Source: CAD feature listing. Evaluate the final solid. Frame: model axes, mm. Face numbers are marked on the shaded views. A direction names the side the tool comes from. Round coordinates to 2 decimals unless told otherwise and drop trailing zeros. Loops run counter-clockwise (first coordinate to the right, second up) from the corner with the lowest first, then second, coordinate; pieces in that order, holes last.
(1) Section C-C, the plane y = -6. Return the cut outline in (x, z), plus the area to 3 significant figures.
(2) Section B-B, the plane x = 42. Return the cut outline in (y, z).
(3) Material intervals for probe 1 along Y at (x, z) = (-63.5, 27.7); probe 2 along Y at (x, z) = (64, 7); probe 3 along Y at (x, z) = (5, 6.5), sorted ascending.
(4) Section D-D, the plane x = 1. Return the cut outline in (y, z).
(5) First-contact query: pin 1 Ø3 at (x, y) = (63, 24.5) entering from +Z; pin 2 Ø3.5 at (x, y) = (-54.5, 26.5) entering from +Z; pin 3 Ø3 at (x, y) = (-8.5, 8) entering from -Z. Flat tips, straight axial feed; report the tip coordinate or a pass-through.
(6) Section A-A, the plane x = -42. Return the cut outline in (y, z), plus the area to 3 significant figures.
(7) Set-up query: the marked faces 4 and 5. Return all of +Z, -Z, +X, -X, +Y, -Y with unobstructed straight access to the full face (end or side cutting, diameter ignored); none if empty.
(8) Mould query, pull axis X, two halves, no side actions, for the marked faces 1, 2 and 3. Classes: pulls with the +X half, pulls with the -X half, needs draft (parallel to the pull), parting line crosses it, or undercut.
```python
from build123d import *

# Parameters (mm, degrees)
SKETCH002_W     = 140
SKETCH002_H     = 66
PAD001_DEPTH    = 4
SKETCH003_W     = 136
SKETCH003_H     = 62
PAD002_DEPTH    = 30
SKETCH004_R     = 3
POCKET001_DEPTH = 5
FILLET_R        = 2
FILLET001_R     = 2
SKETCH005_R     = 1.5
SKETCH005_W     = 10
SKETCH005_H     = 5
POCKET002_DEPTH = 5
SKETCH006_W     = 18
SKETCH006_H     = 9
SKETCH006_W_2   = 9
PAD003_DEPTH    = 6
SKETCH007_W     = 9
SKETCH007_H     = 9
PAD004_DEPTH    = 19
SKETCH008_W     = 9
SKETCH008_H     = 9
PAD005_DEPTH    = 19
SKETCH009_W     = 9
SKETCH009_H     = 9
PAD006_DEPTH    = 25
FILLET004_R     = 1
SKETCH014_W     = 5.5
SKETCH014_H     = 3
POCKET005_DEPTH = 7.5
SKETCH015_W     = 5.5
SKETCH015_H     = 3
POCKET006_DEPTH = 7.5
SKETCH016_W     = 5.5
SKETCH016_H     = 3
POCKET007_DEPTH = 7.4
SKETCH017_W     = 5.5
SKETCH017_H     = 3
POCKET008_DEPTH = 7.5
SKETCH018_W     = 5.5
SKETCH018_H     = 3
POCKET009_DEPTH = 7.5
SKETCH019_W     = 5.5
SKETCH019_H     = 3
POCKET010_DEPTH = 7.5
SKETCH020_R     = 1.6
POCKET011_DEPTH = 12
SKETCH021_R     = 1.6
POCKET012_DEPTH = 12
SKETCH022_R     = 1.6
POCKET013_DEPTH = 12
SKETCH023_R     = 1.6
POCKET014_DEPTH = 12
SKETCH024_R     = 1.6
POCKET015_DEPTH = 8
SKETCH025_R     = 1.6
POCKET016_DEPTH = 8
SKETCH026_R     = 1.6
POCKET017_DEPTH = 8
SKETCH027_R     = 1.6
POCKET018_DEPTH = 8
FILLET005_R     = 1


with BuildPart() as part:
    # Sketch002 → Pad001 (new body)
    with BuildSketch(Plane.XY):
        Rectangle(SKETCH002_W, SKETCH002_H)
    extrude(amount=PAD001_DEPTH)

    # Sketch003 (on Face6 of Pad001) → Pad002 (join)
    with BuildSketch(Plane.XY.offset(4)):
        Polygon((-70, 33), (-70, -33), (-68, -33), (68, -33), (70, -33), (70, 33), (68, 33), (-68, 33), align=None)
        Rectangle(SKETCH003_W, SKETCH003_H, mode=Mode.SUBTRACT)
    extrude(amount=PAD002_DEPTH)

    # Sketch004 (on Face2 of Pad002) → Pocket001 (cut)
    with BuildSketch(Plane.XZ.offset(33)):
        with Locations((42, 25)):
            Circle(SKETCH004_R)
        with Locations((-42, 25)):
            Circle(SKETCH004_R)
        with Locations((-14, 25)):
            Circle(SKETCH004_R)
        with Locations((14, 25)):
            Circle(SKETCH004_R)
    extrude(amount=-POCKET001_DEPTH, mode=Mode.SUBTRACT)

    # Fillet
    fillet_edges = [part.edges().sort_by_distance(p)[0] for p in [
        (-70, -33, 17),
        (70, -33, 17),
    ]]
    fillet(fillet_edges, radius=FILLET_R)

    # Fillet001
    fillet001_edges = [part.edges().sort_by_distance(p)[0] for p in [
        (70, 33, 17),
        (-70, 33, 17),
    ]]
    fillet(fillet001_edges, radius=FILLET001_R)

    # Sketch005 (on Face5 of Fillet001) → Pocket002 (cut)
    with BuildSketch(Plane(origin=(0, 33, 0), x_dir=(-1, 0, 0), z_dir=(0, 1, 0))):
        with Locations((-34.5, 9)):
            Circle(SKETCH005_R)
        with Locations((-51, 9)):
            Circle(SKETCH005_R)
        with Locations((-42.75, 9)):
            Rectangle(SKETCH005_W, SKETCH005_H)
    extrude(amount=-POCKET002_DEPTH, mode=Mode.SUBTRACT)

    # Sketch006 (on Face25 of Pocket002) → Pad003 (join)
    with BuildSketch(Plane.XY.offset(4)):
        with Locations((-59, 26.5)):
            Rectangle(SKETCH006_W, SKETCH006_H)
        with Locations((-59, -26.5)):
            Rectangle(SKETCH006_W, SKETCH006_H)
        with Locations((18.5, 26.5)):
            Rectangle(SKETCH006_W_2, SKETCH006_H)
        with Locations((18.5, -26.5)):
            Rectangle(SKETCH006_W_2, SKETCH006_H)
    extrude(amount=PAD003_DEPTH)

    # Sketch007 (on Face31 of Pad003) → Pad004 (join)
    with BuildSketch(Plane.XY.offset(10)):
        with Locations((-63.5, 26.5)):
            Rectangle(SKETCH007_W, SKETCH007_H)
    extrude(amount=PAD004_DEPTH)

    # Sketch008 (on Face30 of Pad004) → Pad005 (join)
    with BuildSketch(Plane.XY.offset(10)):
        with Locations((-63.5, -26.5)):
            Rectangle(SKETCH008_W, SKETCH008_H)
    extrude(amount=PAD005_DEPTH)

    # Sketch009 (on Face25 of Pad005) → Pad006 (join)
    with BuildSketch(Plane.XY.offset(4)):
        with Locations((63.5, 26.5)):
            Rectangle(SKETCH009_W, SKETCH009_H)
        with Locations((63.5, -26.5)):
            Rectangle(SKETCH009_W, SKETCH009_H)
    extrude(amount=PAD006_DEPTH)

    # Fillet004
    fillet004_edges = [part.edges().sort_by_distance(p)[0] for p in [
        (-68, 31, 31.5),
        (68, 31, 31.5),
        (68, -31, 31.5),
        (-68, -31, 31.5),
    ]]
    fillet(fillet004_edges, radius=FILLET004_R)

    # Sketch014 (on Face36 of Fillet004) → Pocket005 (cut)
    with BuildSketch(Plane.XZ.offset(-22)):
        with Locations((-63.5, 23.5)):
            Rectangle(SKETCH014_W, SKETCH014_H)
        with Locations((-54.5, 6.5)):
            Rectangle(SKETCH014_W, SKETCH014_H)
    extrude(amount=-POCKET005_DEPTH, mode=Mode.SUBTRACT)

    # Sketch015 (on Face33 of Pocket005) → Pocket006 (cut)
    with BuildSketch(Plane.XZ.offset(-22)):
        with Locations((63.5, 23.5)):
            Rectangle(SKETCH015_W, SKETCH015_H)
    extrude(amount=-POCKET006_DEPTH, mode=Mode.SUBTRACT)

    # Sketch016 (on Face35 of Pocket006) → Pocket007 (cut)
    with BuildSketch(Plane(origin=(0, -22, 0), x_dir=(-1, 0, 0), z_dir=(0, 1, 0))):
        with Locations((63.5, 23.5)):
            Rectangle(SKETCH016_W, SKETCH016_H)
        with Locations((54.5, 6.5)):
            Rectangle(SKETCH016_W, SKETCH016_H)
    extrude(amount=-POCKET007_DEPTH, mode=Mode.SUBTRACT)

    # Sketch017 (on Face34 of Pocket007) → Pocket008 (cut)
    with BuildSketch(Plane(origin=(0, -22, 0), x_dir=(-1, 0, 0), z_dir=(0, 1, 0))):
        with Locations((-63.5, 23.5)):
            Rectangle(SKETCH017_W, SKETCH017_H)
    extrude(amount=-POCKET008_DEPTH, mode=Mode.SUBTRACT)

    # Sketch018 (on Face53 of Pocket008) → Pocket009 (cut)
    with BuildSketch(Plane.XZ.offset(-22)):
        with Locations((18.5, 6.5)):
            Rectangle(SKETCH018_W, SKETCH018_H)
    extrude(amount=-POCKET009_DEPTH, mode=Mode.SUBTRACT)

    # Sketch019 (on Face52 of Pocket009) → Pocket010 (cut)
    with BuildSketch(Plane(origin=(0, -22, 0), x_dir=(-1, 0, 0), z_dir=(0, 1, 0))):
        with Locations((-18.5, 6.5)):
            Rectangle(SKETCH019_W, SKETCH019_H)
    extrude(amount=-POCKET010_DEPTH, mode=Mode.SUBTRACT)

    # Sketch020 (on Face37 of Pocket010) → Pocket011 (cut)
    with BuildSketch(Plane.XY.offset(29)):
        with Locations((-63.5, 26.5)):
            Circle(SKETCH020_R)
    extrude(amount=-POCKET011_DEPTH, mode=Mode.SUBTRACT)

    # Sketch021 (on Face18 of Pocket011) → Pocket012 (cut)
    with BuildSketch(Plane.XY.offset(29)):
        with Locations((-63.5, -26.5)):
            Circle(SKETCH021_R)
    extrude(amount=-POCKET012_DEPTH, mode=Mode.SUBTRACT)

    # Sketch022 (on Face32 of Pocket012) → Pocket013 (cut)
    with BuildSketch(Plane.XY.offset(29)):
        with Locations((63.5, 26.5)):
            Circle(SKETCH022_R)
    extrude(amount=-POCKET013_DEPTH, mode=Mode.SUBTRACT)

    # Sketch023 (on Face22 of Pocket013) → Pocket014 (cut)
    with BuildSketch(Plane.XY.offset(29)):
        with Locations((63.5, -26.5)):
            Circle(SKETCH023_R)
    extrude(amount=-POCKET014_DEPTH, mode=Mode.SUBTRACT)

    # Sketch024 (on Face43 of Pocket014) → Pocket015 (cut)
    with BuildSketch(Plane.XY.offset(10)):
        with Locations((-54.5, 26.5)):
            Circle(SKETCH024_R)
    extrude(amount=-POCKET015_DEPTH, mode=Mode.SUBTRACT)

    # Sketch025 (on Face40 of Pocket015) → Pocket016 (cut)
    with BuildSketch(Plane.XY.offset(10)):
        with Locations((18.5, 26.5)):
            Circle(SKETCH025_R)
    extrude(amount=-POCKET016_DEPTH, mode=Mode.SUBTRACT)

    # Sketch026 (on Face26 of Pocket016) → Pocket017 (cut)
    with BuildSketch(Plane.XY.offset(10)):
        with Locations((18.5, -26.5)):
            Circle(SKETCH026_R)
    extrude(amount=-POCKET017_DEPTH, mode=Mode.SUBTRACT)

    # Sketch027 (on Face20 of Pocket017) → Pocket018 (cut)
    with BuildSketch(Plane.XY.offset(10)):
        with Locations((-54.5, -26.5)):
            Circle(SKETCH027_R)
    extrude(amount=-POCKET018_DEPTH, mode=Mode.SUBTRACT)

    # Fillet005
    fillet005_edges = [part.edges().sort_by_distance(p)[0] for p in [
        (68, 22, 16.5),
        (59, 22, 16.5),
        (59, 31, 16.5),
        (23, 31, 7),
        (23, 22, 7),
        (14, 22, 7),
        (14, 31, 7),
        (-68, 22, 16.5),
        (-59, 22, 19.5),
        (-59, 31, 19.5),
        (-50, 22, 7),
        (-50, 31, 7),
        (68, -22, 16.5),
        (59, -22, 16.5),
        (59, -31, 16.5),
        (23, -31, 7),
        (23, -22, 7),
        (14, -22, 7),
        (14, -31, 7),
        (-50, -31, 7),
        (-50, -22, 7),
        (-59, -22, 19.5),
        (-68, -22, 16.5),
        (-59, -31, 19.5),
    ]]
    fillet(fillet005_edges, radius=FILLET005_R)


solid = part.part
```
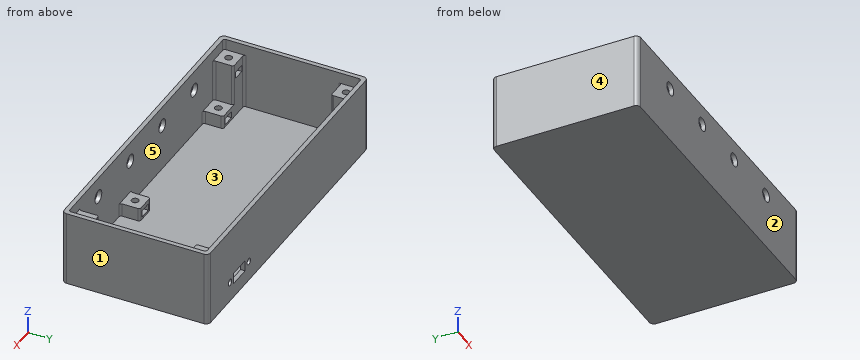
Output values:
1. outline: (-70, 0) - (70, 0) - (70, 34) - (68, 34) - (68, 4) - (-68, 4) - (-68, 34) - (-70, 34) - close
1. area: 680 mm2
2. outline: (-33, 0) - (33, 0) - (33, 6.5) - (31, 6.5) - (31, 4) - (-31, 4) - (-31, 22) - (-33, 22) - close; (-33, 28) - (-31, 28) - (-31, 34) - (-33, 34) - close; (31, 11.5) - (33, 11.5) - (33, 34) - (31, 34) - close
3. probe 1: y = -33 to -28.1, -24.9 to -22, 22 to 24.9, 28.1 to 33
3. probe 2: y = -33 to -22, 22 to 33
3. probe 3: y = -33 to -31, 31 to 33
4. outline: (-33, 0) - (33, 0) - (33, 34) - (31, 34) - (31, 4) - (-31, 4) - (-31, 34) - (-33, 34) - close
5. pin 1: stops at z = 29
5. pin 2: stops at z = 10
5. pin 3: stops at z = 0
6. outline: (-33, 0) - (33, 0) - (33, 34) - (31, 34) - (31, 4) - (-31, 4) - (-31, 22) - (-33, 22) - close; (-33, 28) - (-31, 28) - (-31, 34) - (-33, 34) - close
6. area: 372 mm2
7. face 4: +Z, -Z, -X, +Y, -Y
7. face 5: +Z
8. face 1: pulls with the +X half
8. face 2: needs draft
8. face 3: undercut
